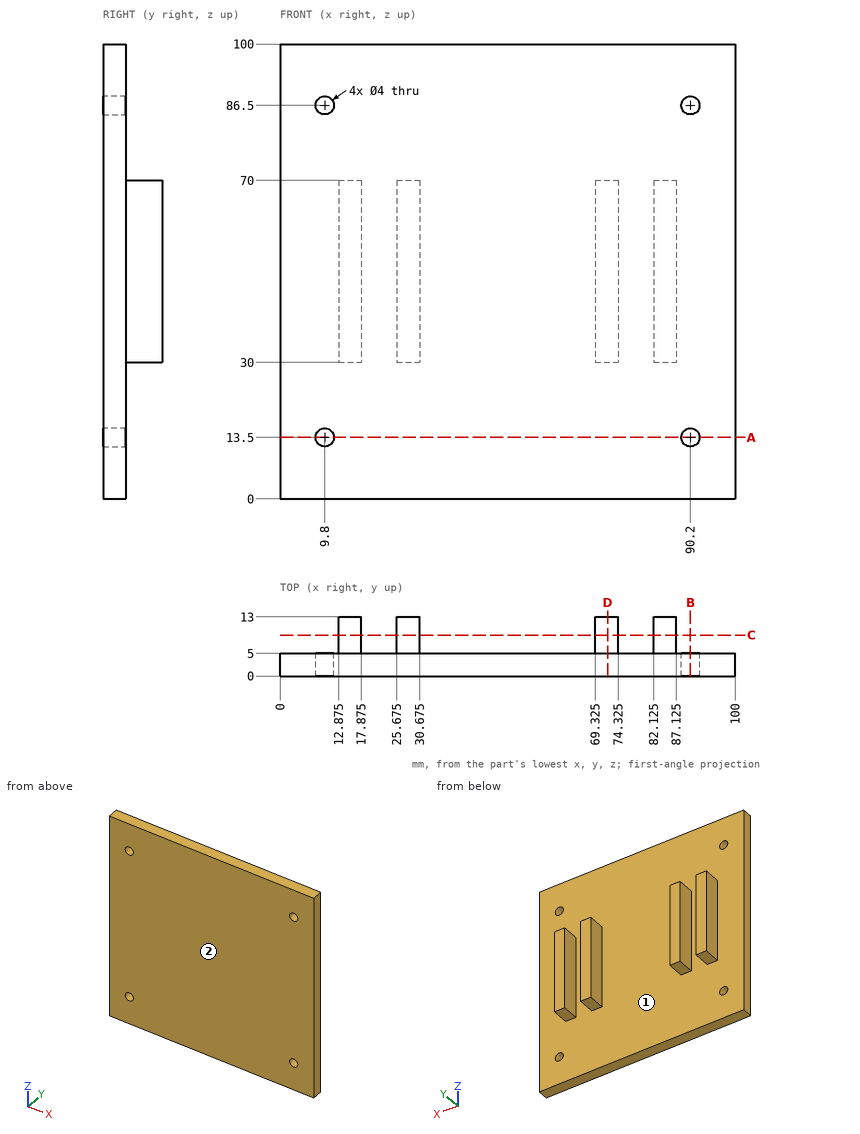
The figure shows three views and two pictorial views of one solid part (mm, origin at its lowest corner). Answer the questions. Coordinates: 2 decimals unless noted, no trailing zeros. Write each loop counter-clockwise with the first axis right and the second up, starting at its lowest first coordinate (ties: lowest second). Pieces come first, ordered by that corner, then holes. Notation, with made-up numbers: M 13,-25 L 19,-25 A22 cw 19,1 Z; hole C 43.25,15.5 d11. An arc over 180 degrees is marked long. Answer as CSV lines item,"result". Start each with the question number.
Item 1: Section C-C on y = 9 is taken. Write down the section's boundary in (x, z) (3 decimals), and give its area (3 significant figures).
Item 2: Section D-D on x = 72 is taken. Write down the section's boundary in (y, z), and give its area (3 significant figures).
Item 3: Flat-ended cylindrical pins translate along their axes: P1, Ø1.5, axis at x = 84, y = 10, coming from the -Z side; P2, Ø4, axis at y = 11, z = 56, coming from the +X side (3 decimals); P3, Ø2, axis at x = 17.5, z = 74.5, coming from the +Y side. Find the tip coordinate at first contact, or state that the pin passes through.
Item 4: Determine the mould class of the marked faces 1 and 2 for opening direction X: released by +X, released by -X, zero draft, split by the parting line, or undercut.
Item 5: Section A-A on z = 13.5 is taken. Write down the section's boundary in (x, y).
Item 6: Section B-B on x = 90.2 is taken. Write down the section's boundary in (y, z), and give its area (3 significant figures).
Item 7: Consider L1, parallel to X at y = 2.05, z = 86.5; L2, parallel to X at y = 7.75, z = 37 (3 decimals); L3, parallel to Y at x = 49, z = 57. Determine where each line is inside the solid, lowest interval first.
Checks:
1,outline,"M 12.875,30 L 17.875,30 L 17.875,70 L 12.875,70 Z; M 25.675,30 L 30.675,30 L 30.675,70 L 25.675,70 Z; M 69.325,30 L 74.325,30 L 74.325,70 L 69.325,70 Z; M 82.125,30 L 87.125,30 L 87.125,70 L 82.125,70 Z"
1,area,"800 mm²"
2,outline,"M 0,0 L 5,0 L 5,30 L 13,30 L 13,70 L 5,70 L 5,100 L 0,100 Z"
2,area,"820 mm²"
3,P1,"stops at z = 30"
3,P2,"stops at x = 87.125"
3,P3,"stops at y = 5"
4,face 1,"undercut"
4,face 2,"zero draft"
5,outline,"M 0,0 L 7.8,0 L 7.8,5 L 0,5 Z; M 11.8,0 L 88.2,0 L 88.2,5 L 11.8,5 Z; M 92.2,0 L 100,0 L 100,5 L 92.2,5 Z"
6,outline,"M 0,0 L 5,0 L 5,11.5 L 0,11.5 Z; M 0,15.5 L 5,15.5 L 5,84.5 L 0,84.5 Z; M 0,88.5 L 5,88.5 L 5,100 L 0,100 Z"
6,area,"460 mm²"
7,L1,"x = 0 to 7.8, 11.8 to 88.2, 92.2 to 100"
7,L2,"x = 12.875 to 17.875, 25.675 to 30.675, 69.325 to 74.325, 82.125 to 87.125"
7,L3,"y = 0 to 5"
